Solid Edge part; units mm, degrees
sketch "Sketch1" plane through (0, 0, 0) normal (0, -1, 0) x (1, 0, 0)
  line L0 (-0.44, 6.6004) -> (0.0279, 8.9147)
  line L1 (0.0279, 8.9147) -> (1.3295, 8.8156)
  line L2 (1.3295, 8.8156) -> (1.4363, 6.4566)
  line L3 (1.4363, 6.4566) -> (3.1967, 5.7909)
  line L4 (3.1967, 5.7909) -> (4.842, 7.4845)
  line L5 (4.842, 7.4845) -> (5.8791, 6.7006)
  line L6 (5.8791, 6.7006) -> (4.6981, 4.6555)
  line L7 (4.6981, 4.6555) -> (5.8186, 3.1435)
  line L8 (5.8186, 3.1435) -> (8.1187, 3.6789)
  line L9 (8.1187, 3.6789) -> (8.5671, 2.4584)
  line L10 (8.5671, 2.4584) -> (6.468, 1.3769)
  line L11 (6.468, 1.3769) -> (6.5896, -0.5008)
  line L12 (6.5896, -0.5008) -> (8.8178, -1.2937)
  line L13 (8.8178, -1.2937) -> (8.5352, -2.5633)
  line L14 (8.5352, -2.5633) -> (6.1844, -2.3383)
  line L15 (6.1844, -2.3383) -> (5.2746, -3.9858)
  line L16 (5.2746, -3.9858) -> (6.7172, -5.8554)
  line L17 (5.7878, -6.7699) -> (6.7172, -5.8554)
  line L18 (5.7878, -6.7699) -> (3.9371, -5.3105)
  line L19 (3.9371, -5.3105) -> (2.2793, -6.2046)
  line L20 (2.2793, -6.2046) -> (2.4841, -8.5573)
  line L21 (1.2122, -8.8277) -> (2.4841, -8.5573)
  line L22 (1.2122, -8.8277) -> (0.4404, -6.5956)
  line L23 (0.4404, -6.5956) -> (-1.437, -6.4523)
  line L24 (-1.437, -6.4523) -> (-2.5378, -8.5415)
  line L25 (-2.5378, -8.5415) -> (-3.7539, -8.0813)
  line L26 (-3.7539, -8.0813) -> (-3.1969, -5.7862)
  line L27 (-3.1969, -5.7862) -> (-4.6979, -4.6514)
  line L28 (-4.6979, -4.6514) -> (-6.7545, -5.813)
  line L29 (-6.7545, -5.813) -> (-7.5283, -4.7685)
  line L30 (-7.5283, -4.7685) -> (-5.819, -3.1393)
  line L31 (-5.819, -3.1393) -> (-6.4682, -1.3724)
  line L32 (-6.4682, -1.3724) -> (-8.8258, -1.2386)
  line L33 (-8.8258, -1.2386) -> (-8.9124, 0.0589)
  line L34 (-8.9124, 0.0589) -> (-6.5933, 0.5052)
  line L35 (-6.5933, 0.5052) -> (-6.1845, 2.3423)
  line L36 (-6.1845, 2.3423) -> (-8.0954, 3.73)
  line L37 (-8.0954, 3.73) -> (-7.4668, 4.8682)
  line L38 (-7.4668, 4.8682) -> (-5.2747, 3.9899)
  line L39 (-5.2747, 3.9899) -> (-3.9375, 5.3144)
  line L40 (-3.9375, 5.3144) -> (-4.796, 7.5158)
  line L41 (-4.796, 7.5158) -> (-3.6515, 8.1347)
  line L42 (-3.6515, 8.1347) -> (-2.2812, 6.2087)
  line L43 (-2.2812, 6.2087) -> (-0.44, 6.6004)
extrude "Protrusion1" add sketch "Sketch1" against normal blind 10
sketch "Sketch2" plane through (0, 0, 0) normal (0, -1, 0) x (1, 0, 0)
  circle A0 centre (0, 0) radius 2.2
extrude "ExtrudedCutout_1" cut sketch "Sketch2" against normal blind 1588.2379
Work out the finished part from the listing and answer in its coordinate system (mm). A direction names the side the tool comes from. Round coordinates to 2 decimals unless told otherwise and drop trailing zeros. Write each loop counter-clockwise with the first axis right and the second up, starting at its lowest first coordinate (ties: lowest second). Pieces come first, ordered by that corner, then holes.
1) Consider probe 1 along X at (y, z) = (7.25, 7); probe 2 along X at (y, z) = (4, 6.75); probe 3 along X at (y, z) = (0.5, -5.25). Determine where each line is inside the solid, lowest interval first.
2) Flat-ended cylindrical pins translate along their axes: P1, Ø1.5, axis at x = -3.5, y = 2, coming from the -Z side; P2, Ø1, axis at y = 5, z = 1, coming from the +X side. Find the tip coordinate at first contact, or state that the pin passes through.
3) Which of the six approach directions +Z, -Z, +X, -X, +Y, -Y give full straight-line access (tool end or side, diameter ignored) to faces 1 (the face through (-7.77, 4.93, 0.28)), 2 (the face through (-5.712, 4.93, -5.224)), 3 (the face through (-2.98, 4.93, 7.19))?
4) A cutting plane is placed at A-A on x = 0.75. Determine the outline of the cut face in (y, z), and give its area (3 significant figures).
5) Determine the mould class of faces 4 (the face through (-6.14, 4.93, -2.27)), 5 (the face through (5.35, 4.93, 7.1)), 6 (the face through (-1.98, 4.93, -7.48)) for opening direction Z: pulls with the +Z half, pulls with the -Z half, needs draft (parallel to the pull), parting line crosses it, or undercut.
Entries:
1. probe 1: x = -4.59 to -2.84, -0.36 to 1.41, 4.37 to 5.48
1. probe 2: x = -4.5 to -2.67, -0.41 to 1.42, 4.13 to 5.81
1. probe 3: x = -7.17 to -5.76, -3.91 to 6.25
2. P1: stops at z = -8.46
2. P2: stops at x = 6.71
3. face 1: -X, +Y, -Y
3. face 2: -Z, +Y, -Y
3. face 3: +Z, +Y, -Y
4. outline: (0, -7.49) - (10, -7.49) - (10, -2.07) - (0, -2.07) - close; (0, 2.07) - (10, 2.07) - (10, 8.86) - (0, 8.86) - close
4. area: 122 mm2
5. face 4: undercut
5. face 5: pulls with the +Z half
5. face 6: pulls with the -Z half
